Geometry check sheet. Reference: the model listing, model coordinates, mm. A direction names the side the tool comes from. Give positions to 0.01 mm unless a question says otherwise; leave off trailing zeros. Write each loop counter-clockwise with the first axis right and the second up, starting at its lowest first coordinate (ties: lowest second). Pieces come first, ordered by that corner, then holes. Notation, with made-up numbers: (36.25, -26.5) - (93.25, -26.5) arc R17 cw to (93.25, -1.5) - close; hole circle Ø10 at (1.5, -16). An arc over 180 degrees is marked (long way). Write item = value, one per line. Start each with the question number.
(1) Section check A-A, the plane z = -21. Enter the section's corners in (x, y), plus the area to 3 significant figures.
(2) Section check B-B, the plane x = 23.55. Enter the section's corners in (y, z).
(3) Access from +Z, -Z, +X, -X, +Y, -Y to the whole of each face (thin tool, end or side, straight path). Record for faces 1 (the cylindrical face through (-22.35, -25.857, -22.916)), 2 (the cylindrical face through (12.932, -5.362, 36.728)), 3 (the flat face through (-7, 13, -45.2)).
(4) Thickness scan on L1, parallel to X at y = -23, z = -9; L2, parallel to Y at x = 0, z = 36. Record the ranges inside material, lowest first.
(5) Draft check along X on faces 4 (the flat face through (-7, 13, 0)), 5 (the flat face through (0, 0, 0)), 6 (the cylindrical face through (23.212, 26.128, -22.916)), 7 (the cylindrical face through (12.932, -5.362, -78.408)). Enter one of: pulls with the +X half, pulls with the -X half, needs draft (parallel to the pull), parting line crosses it, or undercut.
(6) Section check D-D, the plane y = 0. Enter the section's corners in (x, z).
(7) Depth check by flat-ended pin: pin 1 Ø3 at (x, y) = (2, 2.5) entering from +Z; pin 2 Ø12 at (x, z) = (-9.5, -81) entering from +Y; pin 3 Ø7 at (x, y) = (23.55, 23.55) entering from -Z; pin 4 Ø5 at (x, y) = (7.5, -13.5) entering from +Z. Enter the tip coordinate at first touch or a pass-through.
```python
from build123d import *

# Parameters (mm, degrees)
NA23_MOTOR_ENVELOPE_START         = -45.2
SKETCH1_W                         = 56.4
SKETCH1_H                         = 56.4
SKETCH1_R                         = 2.6
NA23_MOTOR_ENVELOPE_DEPTH         = 45.2
REAR_BARREL_ENVELOPE_START        = -110.7
SKETCH2_R                         = 14
REAR_BARREL_ENVELOPE_DEPTH        = 65.5
SKETCH3_R                         = 14
SKETCH3_R_2                       = 5.1
FIXED_FRONT_BARREL_ENVELOPE_DEPTH = 74.5


with BuildPart() as part:
    # Sketch1 → NA23_Motor_Envelope (new body)
    with BuildSketch(Plane.XY.offset(NA23_MOTOR_ENVELOPE_START)):
        Rectangle(SKETCH1_W, SKETCH1_H)
        with Locations((-23.55, -23.55)):
            Circle(SKETCH1_R, mode=Mode.SUBTRACT)
        with Locations((-23.55, 23.55)):
            Circle(SKETCH1_R, mode=Mode.SUBTRACT)
        with Locations((23.55, -23.55)):
            Circle(SKETCH1_R, mode=Mode.SUBTRACT)
        with Locations((23.55, 23.55)):
            Circle(SKETCH1_R, mode=Mode.SUBTRACT)
    extrude(amount=NA23_MOTOR_ENVELOPE_DEPTH)

    # Sketch2 → Rear_Barrel_Envelope (add)
    with BuildSketch(Plane.XY.offset(REAR_BARREL_ENVELOPE_START)):
        Circle(SKETCH2_R)
    extrude(amount=REAR_BARREL_ENVELOPE_DEPTH)

    # Sketch3 → Fixed_Front_Barrel_Envelope (add)
    with BuildSketch(Plane.XY):
        Circle(SKETCH3_R)
        Circle(SKETCH3_R_2, mode=Mode.SUBTRACT)
    extrude(amount=FIXED_FRONT_BARREL_ENVELOPE_DEPTH)


solid = part.part
```
Model answer:
q1.outline = (-28.2, -28.2) - (28.2, -28.2) - (28.2, 28.2) - (-28.2, 28.2) - close; hole circle Ø5.2 at (-23.55, -23.55); hole circle Ø5.2 at (-23.55, 23.55); hole circle Ø5.2 at (23.55, -23.55); hole circle Ø5.2 at (23.55, 23.55)
q1.area = 3,100 mm²
q2.outline = (-28.2, -45.2) - (-26.15, -45.2) - (-26.15, 0) - (-28.2, 0) - close; (-20.95, -45.2) - (20.95, -45.2) - (20.95, 0) - (-20.95, 0) - close; (26.15, -45.2) - (28.2, -45.2) - (28.2, 0) - (26.15, 0) - close
q3.face_1 = +Z, -Z
q3.face_2 = +Z
q3.face_3 = -Z
q4.L1 = -28.2 to -26.09, -21.01 to 21.01, 26.09 to 28.2
q4.L2 = -14 to -5.1, 5.1 to 14
q5.face_4 = needs draft
q5.face_5 = undercut
q5.face_6 = undercut
q5.face_7 = parting line crosses it
q6.outline = (-28.2, -45.2) - (-14, -45.2) - (-14, -110.7) - (14, -110.7) - (14, -45.2) - (28.2, -45.2) - (28.2, 0) - (14, 0) - (14, 74.5) - (5.1, 74.5) - (5.1, 0) - (-5.1, 0) - (-5.1, 74.5) - (-14, 74.5) - (-14, 0) - (-28.2, 0) - close
q7.pin_1 = 0
q7.pin_2 = 13.56
q7.pin_3 = -45.2
q7.pin_4 = 74.5
